Part model, mm, in its own coordinate system. A direction names the side the tool comes from. Round coordinates to 2 decimals unless told otherwise and drop trailing zeros. Order: outer loops, then holes, each group sorted by start corner. A loop starts at its lowest first (then second) coordinate and runs counter-clockwise, first axis right, second up. Notation, with made-up numbers: (-23, 16) -> (4, 16) arc R14 cw to (4, 34) -> close; hole circle Ø9 at (-4, 46). An arc over 180 degrees is marked (long way). Answer as a JSON object with one key per item and string values. Group by question number.
Autodesk Inventor part; units mm, degrees
ref_plane "YZ Plane" through (0, 0, 0) normal (1, 0, 0) x (0, 1, 0)
ref_plane "XZ Plane" through (0, 0, 0) normal (0, 1, 0) x (-1, 0, 0)
ref_plane "XY Plane" through (0, 0, 0) normal (0, 0, 1) x (1, 0, 0)
sketch "Sketch1" plane through (0, 0, 0) normal (0, 0, 1) x (1, 0, 0)
  line L0 (-46.5, 43.5) -> (46.5, 43.5)
  line L1 (46.5, 43.5) -> (46.5, -43.5)
  line L2 (46.5, -43.5) -> (-46.5, -43.5)
  line L3 (-46.5, -43.5) -> (-46.5, 43.5)
  point P0 (0, 0)
  dimension "d0" = 93
  dimension "d1" = 87
  dimension "d2" = 46.5
  dimension "d3" = 43.5
extrude "Tykkelse Rød PCB" add sketch "Sketch1" along normal blind 1.5
sketch "Sketch2" plane through (0, 0, 1.5) normal (0, 0, 1) x (1, 0, 0)
  line L0 (46.5, 43.5) -> (-46.5, 43.5)
  line L1 (-46.5, 43.5) -> (-46.5, -43.5)
  line L2 (46.5, -43.5) -> (46.5, 43.5)
  circle A0 centre (44, 41) radius 1.5
  circle A1 centre (-44, 41) radius 1.5
  line L3 (45.5, 42.5) -> (45.5, 26.8687) construction
  line L4 (4.2035, 42.5) -> (45.5, 42.5) construction
  line L5 (-45.5, 42.5) -> (-9.5739, 42.5) construction
  line L6 (-45.5, 42.5) -> (-45.5, 29.332) construction
  line L7 (-46.5, -43.5) -> (46.5, -43.5)
  circle A2 centre (-44, -24) radius 1.5
  circle A3 centre (44, -24) radius 1.5
  line L8 (45.5, -14.3819) -> (45.5, -25.5) construction
  line L9 (45.5, -25.5) -> (38.4616, -25.5) construction
  line L10 (-45.5, -14.3819) -> (-45.5, -25.5) construction
  line L11 (-36.8227, -25.5) -> (-45.5, -25.5) construction
  point P0 (0, 0)
  dimension "d6" = 3
  dimension "d7" = 3
  dimension "d8" = 1
  dimension "d9" = 1
  dimension "d10" = 1
  dimension "d11" = 1
  dimension "d79" = 1
  dimension "d80" = 3
  dimension "d81" = 65
  dimension "d82" = 3
  dimension "d83" = 1
  dimension "d84" = 65
extrude "Monteringshuller Ø3" cut sketch "Sketch2" against normal up to surface (1.5 mm away) contours A0 | A1 | A2 | A3
sketch "Sketch3" plane through (0, 0, 0) normal (0, 0, -1) x (-1, 0, 0)
  line L0 (46.5, 43.5) -> (-46.5, 43.5)
  line L1 (-46.5, 43.5) -> (-46.5, -43.5)
  line L2 (46.5, -43.5) -> (46.5, 43.5)
  line L3 (-25.5, 37.5) -> (-5.5, 37.5)
  line L4 (-5.5, 37.5) -> (-5.5, 28.5)
  line L5 (-5.5, 28.5) -> (-25.5, 28.5)
  line L6 (-25.5, 28.5) -> (-25.5, 37.5)
  line L7 (5.5, 37.5) -> (25.5, 37.5)
  line L8 (25.5, 37.5) -> (25.5, 28.5)
  line L9 (25.5, 28.5) -> (5.5, 28.5)
  line L10 (5.5, 28.5) -> (5.5, 37.5)
  point P0 (0, 0)
  dimension "d14" = 20
  dimension "d15" = 9
  dimension "d16" = 9
  dimension "d17" = 20
  dimension "d18" = 21
  dimension "d19" = 21
  dimension "d20" = 6
  dimension "d21" = 6
extrude "Sorte Stik" add sketch "Sketch3" along normal blind 9
sketch "Sketch4" plane through (0, 0, 0) normal (0, 0, -1) x (-1, 0, 0)
  line L0 (46.5, 43.5) -> (-46.5, 43.5)
  line L1 (46.5, -43.5) -> (46.5, 43.5)
  line L2 (25.5, 21.5) -> (46.5, 21.5)
  line L3 (46.5, 21.5) -> (46.5, -0.5)
  line L4 (46.5, -0.5) -> (25.5, -0.5)
  line L5 (25.5, -0.5) -> (25.5, 21.5)
  point P0 (0, 0)
  dimension "d24" = 22
  dimension "d25" = 21
  dimension "d26" = 0
  dimension "d27" = 22
extrude "SD Kort læser" add sketch "Sketch4" along normal blind 4
sketch "Sketch5" plane through (0, 0, 1.5) normal (0, 0, 1) x (1, 0, 0)
  line L0 (-46.5, -43.5) -> (46.5, -43.5)
  line L1 (46.5, -43.5) -> (46.5, 43.5)
  line L2 (43.5, -29) -> (30, -29)
  line L3 (30, -29) -> (30, -41.5)
  line L4 (30, -41.5) -> (43.5, -41.5)
  line L5 (43.5, -41.5) -> (43.5, -29)
  point P0 (0, 0)
  dimension "d30" = 12.5
  dimension "d31" = 13.5
  dimension "d32" = 3
  dimension "d33" = 2
extrude "Extrusion5" add sketch "Sketch5" along normal blind 6
sketch "Sketch6" plane through (0, 0, 7.5) normal (0, 0, 1) x (1, 0, 0)
  line L0 (43.5, -29) -> (30, -29)
  line L1 (30, -29) -> (30, -41.5)
  line L2 (30, -41.5) -> (43.5, -41.5)
  circle A0 centre (36.75, -35.25) radius 6.25
  point P0 (0, 0)
  dimension "d36" = 6.75
  dimension "d37" = 13.5
extrude "Extrusion6" add sketch "Sketch6" along normal blind 19 contours A0
chamfer "Chamfer1" distance 1 angle 45 1 edges at (30.5, -35.25, 26.5)
sketch "Sketch7" plane through (0, 0, 1.5) normal (0, 0, 1) x (1, 0, 0)
  line L0 (-46.5, -43.5) -> (46.5, -43.5)
  line L1 (46.5, -43.5) -> (46.5, 43.5)
  circle A0 centre (19.75, -34.75) radius 5.75
  line L2 (25.5, -40.5) -> (6.0957, -40.5) construction
  line L3 (25.5, -23.1538) -> (25.5, -40.5) construction
  point P0 (0, 0)
  dimension "d43" = 11.5
  dimension "d44" = 3
  dimension "d45" = 21
extrude "Extrusion7" add sketch "Sketch7" along normal blind 9
sketch "Sketch8" plane through (19.75, -34.75, 10.5) normal (0, 0, 1) x (1, 0, 0)
  circle A0 centre (0, 0) radius 5.75
  circle A1 centre (0, 0) radius 1
  point P0 (-19.75, 34.75)
  dimension "d48" = 2
extrude "Extrusion8" cut sketch "Sketch8" against normal blind 4 contours A1
sketch "Sketch9" plane through (0, 0, 1.5) normal (0, 0, 1) x (1, 0, 0)
  line L0 (-46.5, -43.5) -> (46.5, -43.5)
  line L1 (46.5, -43.5) -> (46.5, 43.5)
  line L2 (0.5, -32.5) -> (6.5, -32.5)
  line L3 (6.5, -32.5) -> (6.5, -38.5)
  line L4 (6.5, -38.5) -> (0.5, -38.5)
  line L5 (0.5, -38.5) -> (0.5, -32.5)
  point P0 (0, 0)
  dimension "d51" = 6
  dimension "d52" = 6
  dimension "d53" = 5
  dimension "d54" = 40
extrude "Extrusion9" add sketch "Sketch9" along normal blind 4
sketch "Sketch10" plane through (0, 0, 5.5) normal (0, 0, 1) x (1, 0, 0)
  line L0 (6.5, -32.5) -> (0.5, -32.5)
  line L1 (6.5, -38.5) -> (6.5, -32.5)
  circle A0 centre (3.5, -35.5) radius 1.5
  point P0 (0, 0)
  dimension "d57" = 3
  dimension "d58" = 6
  dimension "d59" = 6
  dimension "d60" = 3
  dimension "d61" = 3
extrude "Extrusion10" add sketch "Sketch10" along normal blind 3
fillet "Fillet1" radius 0.5 1 edges at (2, -35.5, 8.5)
fillet "Fillet2" radius 0.5 1 edges at (14, -34.75, 10.5)
sketch "Sketch11" plane through (36.75, -35.25, 26.5) normal (0, 0, 1) x (1, 0, 0)
  circle A0 centre (0, 0) radius 5.25
  line L0 (0, 0) -> (0, -4.739) construction
  line L1 (0, 0) -> (-2.5895, -4.4851) construction
  line L2 (-2.089, -3.1183) -> (-3.339, -5.2833)
  line L3 (-2.089, -3.1183) -> (-1.656, -3.3683)
  circle A1 centre (0, 0) radius 6.25
  circle A2 centre (0, 0) radius 5.25
  line L4 (-2.906, -5.5333) -> (-1.656, -3.3683)
  point P0 (-36.75, 35.25)
  dimension "d66" = 30
  dimension "d68" = 0.25
  dimension "d69" = 2.5
  dimension "d70" = 0.5
extrude "Extrusion11" cut sketch "Sketch11" against normal blind 1 contours L2 L3 L4 A0 | A0 L4 A1 L2 picked at (-2.0992, -3.6914) picked at (-2.6213, -4.9292)
sketch "Sketch12" plane through (-46.5, -43.5, 1.5) normal (-1, 0, 0) x (0, 0, 1)
  line L0 (-1.5, 65) -> (-1.5, 87)
  line L1 (-1.5, 65) -> (-5.5, 65)
  line L2 (-5.5, 43) -> (-5.5, 65)
  line L3 (-1.5, 43) -> (-5.5, 43)
  line L4 (-4.5, 64) -> (-1.5, 64)
  line L5 (-1.5, 64) -> (-1.5, 44)
  line L6 (-1.5, 44) -> (-4.5, 44)
  line L7 (-4.5, 44) -> (-4.5, 64)
  point P0 (-1.5, 43.5)
  dimension "d73" = 1
  dimension "d74" = 1
  dimension "d75" = 1
  dimension "d76" = 0
extrude "Extrusion12" add sketch "Sketch12" along normal blind 10
sketch "Sketch13" plane through (0, 0, 26.5) normal (0, 0, 1) x (1, 0, 0)
  arc A0 (-34.5, 28.5) -> (-36.5, 26.5) centre (-34.5, 26.5) ccw
  line L0 (-34.5, 28.5) -> (34.5, 28.5)
  arc A1 (36.5, 26.5) -> (34.5, 28.5) centre (34.5, 26.5) ccw
  line L1 (36.5, 26.5) -> (36.5, -8.5)
  arc A2 (34.5, -10.5) -> (36.5, -8.5) centre (34.5, -8.5) ccw
  line L2 (34.5, -10.5) -> (-34.5, -10.5)
  arc A3 (-36.5, -8.5) -> (-34.5, -10.5) centre (-34.5, -8.5) ccw
  line L3 (-36.5, -8.5) -> (-36.5, 26.5)
  line L4 (39, 34.5) -> (-39, 34.5)
  line L5 (-39, 34.5) -> (-39, -16.5)
  line L6 (-39, -16.5) -> (39, -16.5)
  line L7 (39, -16.5) -> (39, 34.5)
  line L8 (-39, 30.5) -> (-39, -11.5)
  line L9 (-39, 30.5) -> (-45.5, 30.5)
  line L10 (-45.5, 30.5) -> (-45.5, -11.5)
  line L11 (-45.5, -11.5) -> (-39, -11.5)
  circle A4 centre (3.5, -35.5) radius 1.5
  circle A5 centre (19.75, -34.75) radius 5.75
  arc A6 (33.844, -40.7833) -> (33.411, -40.5333) centre (36.75, -35.25) ccw
  line L12 (-34.5, 26.5) -> (34.5, -8.5) construction
  line L13 (34.5, 26.5) -> (-34.5, -8.5) construction
  line L14 (0, 28.5) -> (0, 9) construction
  point P0 (0, 0)
  dimension "d85" = 36.75
  dimension "d86" = 6.25
  dimension "d87" = 11.5
  dimension "d88" = 19.75
  dimension "d89" = 3
  dimension "d90" = 3.5
  dimension "d91" = 44.5
  dimension "d92" = 43.75
  dimension "d93" = 44.25
equation "\"d16\" = d15"
equation "\"d17\" = d14"
equation "\"d19\" = d18"
equation "\"d21\" = d20"
equation "\"d36\" = 0.5 * d37"
equation "\"d60\" = 0.5 * d58"
equation "\"d61\" = 0.5 * d59"
equation "\"d68\" = 0.5 * d70"
properties part number "Rød PCB"
Q1. Two-plate mould, pull along X, no slides. Class faces 5 (the flat face through (-16, 28.5, -4)), 6 (the cylindrical face through (-45.11, -22.99, 0.76)): +X half, -X half, draft (parallel to the pull), parting line (faces both ways), or undercut.
Q2. Which spindle directions (+Z, -Z, +X, -X, +Y, -Y) get a long thin tool onto all of the face, cutting with end or side? Do faces 1 (the flat face through (30, -35, 4)), 2 (the flat face through (-51, 20.5, -2)), 3 (the flat face through (-51, 0.5, -1)), 4 (the cylindrical face through (35.936, -41.447, 16.374)). Say none if no direction does.
Q3. Wall check: line 1 (Y direction, x = 44, z = 1.1); line 2 (Y direction, x = 19.75, z = 7.8); line 3 (X direction, y = -34, z = 9). Give the ranges that are in metal, low to high. Write a range as [from, to].
Q4. Band-saw the part on D-D (y = 35.5). List the corners of the cut face in (x, z), plus the area to 4 significant figures.
Q5. Band-saw the part on B-B (z = 4). List the corners of the cut face in (x, y), plus the area to 3 significant figures.
Q6. Band-saw the part on A-A (z = -5.5). List the corners of the cut face in (x, y), plus the area to 3 significant figures.
Q7. Band-saw the part on C-C (y = -24). List the corners of the cut face in (x, z).
Q8. Drop flat-ended pins along their axis: pin 1 Ø10 at (x, z) = (17, -5.5) entering from -Y; pin 2 Ø12 at (x, z) = (5.5, 8) entering from -Y; pin 3 Ø1.2 at (x, z) = (3.5, 3.5) entering from +Y; pin 4 Ø1.5 at (x, z) = (-43.5, 2.5) entering from +Y. Give the stop position or say it passes through.
Completed:
{
 "1": {"face 5": "draft", "face 6": "undercut"},
 "2": {"face 1": "+Z, +Y, -Y", "face 2": "+Z, -Z, -X, +Y", "face 3": "+Z, -Z, -X, -Y", "face 4": "+Z"},
 "3": {"line 1": "[-43.5, -25.5], [-22.5, 39.5], [42.5, 43.5]", "line 2": "[-40.5, -35.75], [-33.75, -29]", "line 3": "[14.05, 19.09], [20.41, 25.45], [30.63, 42.87]"},
 "4": {"outline": "(-46.5, 0) -> (-25.5, 0) -> (-25.5, -9) -> (-5.5, -9) -> (-5.5, 0) -> (5.5, 0) -> (5.5, -9) -> (25.5, -9) -> (25.5, 0) -> (46.5, 0) -> (46.5, 1.5) -> (-46.5, 1.5) -> close", "area": "499.5 mm2"},
 "5": {"outline": "(0.5, -38.5) -> (6.5, -38.5) -> (6.5, -32.5) -> (0.5, -32.5) -> close; circle Ø11.5 at (19.75, -34.75); (30, -41.5) -> (43.5, -41.5) -> (43.5, -29) -> (30, -29) -> close", "area": "309 mm2"},
 "6": {"outline": "(-25.5, 28.5) -> (-5.5, 28.5) -> (-5.5, 37.5) -> (-25.5, 37.5) -> close; (5.5, 28.5) -> (25.5, 28.5) -> (25.5, 37.5) -> (5.5, 37.5) -> close", "area": "360 mm2"},
 "7": {"outline": "(-46.5, 0) -> (-45.5, 0) -> (-45.5, 1.5) -> (-46.5, 1.5) -> close; (-42.5, 0) -> (42.5, 0) -> (42.5, 1.5) -> (-42.5, 1.5) -> close; (45.5, 0) -> (46.5, 0) -> (46.5, 1.5) -> (45.5, 1.5) -> close"},
 "8": {"pin 1": "y = 28.5", "pin 2": "y = -38.5", "pin 3": "y = -32.5", "pin 4": "through"}
}
